```python
from build123d import *

# Parameters (mm, degrees)
SKETCH073_R     = 1.698831
PAD043_DEPTH    = 4
SKETCH074_W     = 15
SKETCH074_H     = 15
PAD044_DEPTH    = 6.5
SKETCH078_W     = 4
SKETCH078_H     = 4
POCKET033_DEPTH = 6
FILLET006_R     = 1
POCKET047_DEPTH = 7


with BuildPart() as part:
    # Sketch073 → Pad043 (new body)
    with BuildSketch(Plane(origin=(0, 0, 25), x_dir=(1, 0, 0), z_dir=(0, 0, -1))):
        with Locations((5.5, 22.5)):
            Circle(SKETCH073_R)
    extrude(amount=-PAD043_DEPTH)

    # Sketch074 (on Face2 of Pad043) → Pad044 (join)
    with BuildSketch(Plane(origin=(0, 0, 25), x_dir=(1, 0, 0), z_dir=(0, 0, -1))):
        with Locations((5.5, 22.5)):
            Rectangle(SKETCH074_W, SKETCH074_H)
    extrude(amount=PAD044_DEPTH)

    # Sketch078 → Pocket033 (cut)
    with BuildSketch(Plane(origin=(0, 0, 18.5), x_dir=(1, 0, 0), z_dir=(0, 0, -1))):
        with Locations((5.5, 22.5)):
            Rectangle(SKETCH078_W, SKETCH078_H)
    extrude(amount=-POCKET033_DEPTH, mode=Mode.SUBTRACT)

    # Fillet006
    fillet006_edges = [part.edges().sort_by_distance(p)[0] for p in [
        (13, -30, 21.75),
        (13, -15, 21.75),
        (-2, -15, 21.75),
        (-2, -30, 21.75),
    ]]
    fillet(fillet006_edges, radius=FILLET006_R)

    # Sketch096 (on Face5 of Fillet006) → Pocket047 (cut)
    with BuildSketch(Plane(origin=(0, 0, 18.5), x_dir=(1, 0, 0), z_dir=(0, 0, -1))):
        Polygon((3, 27), (8, 27), (9, 30), (2, 30), align=None)
        Polygon((1, 25), (-2, 26), (-2, 19), (1, 20), align=None)
        Polygon((3, 18), (2, 15), (9, 15), (8, 18), align=None)
        Polygon((10, 25), (13, 26), (13, 19), (10, 20), align=None)
    extrude(amount=-POCKET047_DEPTH, mode=Mode.SUBTRACT)


with BuildPart() as part_1:
    # Body007 placement: moved
    add(part.part.moved(Location((0, 0, 4))))


solid = part_1.part
```
Verification items for the finished model (mm, model axes). A direction names the side the tool comes from. Coordinates: 2 decimals unless noted, no trailing zeros. Loops run counter-clockwise (first coordinate to the right, second up) from the corner with the lowest first, then second, coordinate; pieces in that order, holes last. Notation, with made-up numbers: (11, 22) -> (53, 22) arc R28 ccw to (53, 41) -> close; hole circle Ø3 at (79.25, 83.25). An arc over 180 degrees is marked (long way). Answer in a Markdown table with one row per item. Add a question column.
1. Section check D-D, the plane y = -22.5. Enter the section's corners in (x, z), then the cut area to 3 significant figures.
2. Section check C-C, the plane x = 5.5. Enter the section's corners in (y, z).
3. Section check A-A, the plane z = 28. Enter the section's corners in (x, y), then the cut area to 3 significant figures.
4. Draft check along Y on faces 1 (the face through (11.5, -25.5, 25.7)), 2 (the face through (8.5, -16.5, 25.7)), 3 (the face through (5.279, -24.184, 30.972)). Enter one of: +Y half, -Y half, draft (parallel to the pull), parting line (faces both ways), or undercut.
5. Material ranges on probe 1 along X at (y, z) = (-23.5, 24); probe 2 along Z at (x, y) = (-1, -17.5); probe 3 along Y at (x, z) = (7.75, 25), recorded low to high. Write a range as [from, to].
6. Section check B-B, the plane x = 0.25. Enter the section's corners in (y, z), then the cut area to 4 significant figures.
7. Access from +Z, -Z, +X, -X, +Y, -Y to the whole of each face (thin tool, end or side, straight path). Record for faces 4 (the face through (10, -22, 26)), 5 (the face through (7.5, -22, 25)), 6 (the face through (2.5, -16.5, 25.7)).
8. Depth check by flat-ended pin: P1, Ø1.2, axis at y = -22.5, z = 24, coming from the -X side; P2, Ø2, axis at x = 6.5, z = 26.5, coming from the -Y side; P3, Ø5, axis at x = 11.5, y = -27.5, coming from the +Z side. Enter the tip coordinate at first touch or a pass-through.
Derived:
| question | item | result |
|---|---|---|
| 1 | outline | (1, 22.5) -> (3.5, 22.5) -> (3.5, 28.5) -> (7.5, 28.5) -> (7.5, 22.5) -> (10, 22.5) -> (10, 29) -> (7.2, 29) -> (7.2, 33) -> (3.8, 33) -> (3.8, 29) -> (1, 29) -> close |
| 1 | area | 48.1 mm² |
| 2 | outline | (-27, 22.5) -> (-24.5, 22.5) -> (-24.5, 28.5) -> (-20.5, 28.5) -> (-20.5, 22.5) -> (-18, 22.5) -> (-18, 29) -> (-20.8, 29) -> (-20.8, 33) -> (-24.2, 33) -> (-24.2, 29) -> (-27, 29) -> close |
| 3 | outline | (-2, -29) arc R1 ccw to (-1, -30) -> (2, -30) -> (3, -27) -> (8, -27) -> (9, -30) -> (12, -30) arc R1 ccw to (13, -29) -> (13, -26) -> (10, -25) -> (10, -20) -> (13, -19) -> (13, -16) arc R1 ccw to (12, -15) -> (9, -15) -> (8, -18) -> (3, -18) -> (2, -15) -> (-1, -15) arc R1 ccw to (-2, -16) -> (-2, -19) -> (1, -20) -> (1, -25) -> (-2, -26) -> close; hole (3.5, -24.5) -> (7.5, -24.5) -> (7.5, -20.5) -> (3.5, -20.5) -> close |
| 3 | area | 136 mm² |
| 4 | face 1 | undercut |
| 4 | face 2 | +Y half |
| 4 | face 3 | parting line |
| 5 | probe 1 | x = [1, 3.5], [7.5, 10] |
| 5 | probe 2 | z = [22.5, 29] |
| 5 | probe 3 | y = [-27, -18] |
| 6 | outline | (-30, 22.5) -> (-25.25, 22.5) -> (-25.25, 29) -> (-30, 29) -> close; (-19.75, 22.5) -> (-15, 22.5) -> (-15, 29) -> (-19.75, 29) -> close |
| 6 | area | 61.75 mm² |
| 7 | face 4 | +Z, -Z, +X |
| 7 | face 5 | -Z |
| 7 | face 6 | +Z, -Z, +Y |
| 8 | P1 | stops at x = 1 |
| 8 | P2 | stops at y = -27 |
| 8 | P3 | stops at z = 29 |
